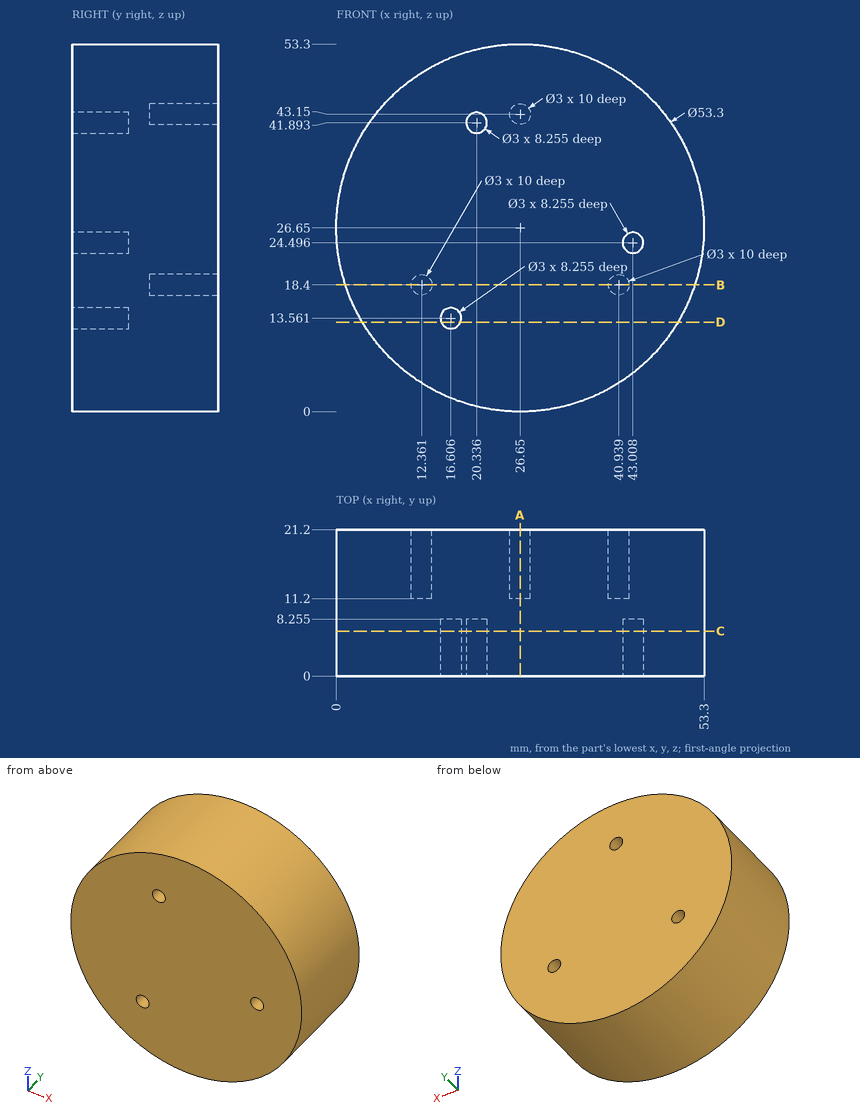
Here's the drawing with two shaded views (mm, measured from the low corner). I have some questions. Give positions to 0.01 mm unless a question says otherwise; leave off trailing zeros. Order: outer loops, then holes, each group sorted by start corner. A loop starts at its lowest first (then second) coordinate and runs counter-clockwise, first axis right, second up. Notation, with made-up numbers: M 23.5,-9 L 65.5,-9 A17 cw 65.5,9 Z; hole C 22,37.5 d9. An arc over 180 degrees is marked long. Answer as a JSON object with one key per item and string values. Group by question number.
1) Suppose I cut it at D-D, the plane z = 13. Write out the boundary of the cut face in (x, y) (1 decimal).
2) Please list where these lines run through material, in increasing order: L1, parallel to X at y = 16.5, z = 18.4; L2, parallel to X at y = 18.5, z = 19.5 (1 decimal); L3, parallel to X at y = 18.75, z = 42 (1 decimal). Write a range as [from, to].
3) Suppose I cut it at B-B, the plane z = 18.4. Write out the boundary of the cut face in (x, y), plus the area to 3 significant figures.
4) I'm going to push flat-ended pins straight in: pin 1 Ø1.5 at (x, z) = (16, 13.5) entering from -Y (3 decimals); pin 2 Ø1.5 at (x, z) = (40.5, 18.5) entering from +Y; pin 3 Ø3 at (y, z) = (17, 16) entering from -X; pin 4 Ø2.5 at (x, z) = (40.94, 18.4) entering from -Y. Where does each tip first touch, or does it pass through?
5) Suppose I cut it at A-A, the plane x = 26.65. Write out the boundary of the cut face in (y, z), plus the area to 3 significant figures.
6) Suppose I cut it at C-C, the plane y = 6.5. Write out the boundary of the cut face in (x, z), plus the area to 3 significant figures.
Results found:
{
 "1": {"outline": "M 3.8,0 L 15.2,0 L 15.2,8.3 L 18,8.3 L 18,0 L 49.5,0 L 49.5,21.2 L 3.8,21.2 Z"},
 "2": {"L1": "[1.31, 10.86], [13.86, 39.44], [42.44, 51.99]", "L2": "[1, 11.3], [13.4, 39.9], [42, 52.3]", "L3": "[4.9, 25.7], [27.6, 48.4]"},
 "3": {"outline": "M 1.31,0 L 51.99,0 L 51.99,21.2 L 42.44,21.2 L 42.44,11.2 L 39.44,11.2 L 39.44,21.2 L 13.86,21.2 L 13.86,11.2 L 10.86,11.2 L 10.86,21.2 L 1.31,21.2 Z", "area": "1,010 mm²"},
 "4": {"pin 1": "y = 8.255", "pin 2": "y = 11.2", "pin 3": "x = 1.62", "pin 4": "y = 0"},
 "5": {"outline": "M 0,0 L 21.2,0 L 21.2,41.65 L 11.2,41.65 L 11.2,44.65 L 21.2,44.65 L 21.2,53.3 L 0,53.3 Z", "area": "1,100 mm²"},
 "6": {"outline": "C 26.65,26.65 d53.3; hole C 16.61,13.56 d3; hole C 20.34,41.89 d3; hole C 43.01,24.5 d3", "area": "2,210 mm²"}
}
